```python
from build123d import *

# Parameters (mm, degrees)
SKETCH1_W               = 7
SKETCH1_H               = 15
BOSS_EXTRUDE1_DEPTH     = 9
SKETCH2_R               = 4.5
CUT_EXTRUDE1_DEPTH      = 14.647344064
CUT_EXTRUDE2_DEPTH      = 2.1
CUT_EXTRUDE2_DEPTH_BACK = 2.1
SKETCH3_R               = 6.1
FILLET1_R               = 7.5
BOSS_EXTRUDE2_DEPTH     = 4
SKETCH5_R               = 1.75
CUT_EXTRUDE3_DEPTH      = 17.194134741


with BuildPart() as part:
    # Sketch1 → Boss-Extrude1 (new body)
    with BuildSketch(Plane.XY):
        Rectangle(SKETCH1_W, SKETCH1_H)
    extrude(amount=BOSS_EXTRUDE1_DEPTH)

    # Sketch2 → Cut-Extrude1 (cut, through all)
    with BuildSketch(Plane(origin=(3.5, 0, 0), x_dir=(0, 0, -1), z_dir=(1, 0, 0))):
        Circle(SKETCH2_R)
    extrude(amount=-CUT_EXTRUDE1_DEPTH, mode=Mode.SUBTRACT)

    # Sketch3 → Cut-Extrude2 (cut, two sides: drawn at the far end of the back side and taken through both)
    with BuildSketch(Plane(origin=(0, 0, 0), x_dir=(0, 0, -1), z_dir=(1, 0, 0)).offset(-CUT_EXTRUDE2_DEPTH_BACK)):
        Circle(SKETCH3_R)
    extrude(amount=CUT_EXTRUDE2_DEPTH + CUT_EXTRUDE2_DEPTH_BACK, mode=Mode.SUBTRACT)

    # Fillet1
    fillet1_edges = [part.edges().sort_by_distance(p)[0] for p in [
        (0, -7.5, 9),
        (0, 7.5, 9),
    ]]
    fillet(fillet1_edges, radius=FILLET1_R - 0.0001)  # a hair under: the kernel refuses the full size

    # Sketch4 → Boss-Extrude2 (add)
    with BuildSketch(Plane.XY):
        with BuildLine():
            Line((-3.5, 6.507281557), (-3.5, 9.5))
            ThreePointArc((-3.5, 9.5), (0, 13), (3.5, 9.5))
            Line((3.5, 9.5), (3.5, 6.507281557))
            Line((3.5, 6.507281557), (-3.5, 6.507281557))
        make_face()
    boss_extrude2 = extrude(amount=BOSS_EXTRUDE2_DEPTH)

    # Sketch5 → Cut-Extrude3 (cut, through all)
    with BuildSketch(Plane(origin=(0, 0, 0), x_dir=(-1, 0, 0), z_dir=(0, 0, -1))):
        with Locations((0, 10)):
            Circle(SKETCH5_R)
    cut_extrude3 = extrude(amount=-CUT_EXTRUDE3_DEPTH, mode=Mode.SUBTRACT)

    # Mirror1: Boss-Extrude2, Cut-Extrude3 across plane
    add(boss_extrude2.mirror(Plane.ZX))
    add(cut_extrude3.mirror(Plane.ZX), mode=Mode.SUBTRACT)


solid = part.part
```
Verification items for the finished model (mm, model axes). A direction names the side the tool comes from. Round coordinates to 2 decimals unless told otherwise and drop trailing zeros. Order: outer loops, then holes, each group sorted by start corner. A loop starts at its lowest first (then second) coordinate and runs counter-clockwise, first axis right, second up.
1) Cross-section at A-A, the plane x = 0. Give the number of separate pieces and of enclosed holes in the cut face, plus the area to 3 significant figures.
Geometry says:
separate pieces: 3
enclosed holes: 0
area: 69.1 mm2
2) Cross-section at B-B, the plane z = 3.25. Record the cut outline in (x, y).
Geometry says:
outline: (-3.5, -9.5) arc R3.5 ccw to (3.5, -9.5) - (3.5, -3.11) - (2.1, -3.11) - (2.1, -5.16) - (-2.1, -5.16) - (-2.1, -3.11) - (-3.5, -3.11) - close; (-3.5, 3.11) - (-2.1, 3.11) - (-2.1, 5.16) - (2.1, 5.16) - (2.1, 3.11) - (3.5, 3.11) - (3.5, 9.5) arc R3.5 ccw to (-3.5, 9.5) - close; hole circle Ø3.5 at (0, -10); hole circle Ø3.5 at (0, 10)
3) Depth check by flat-ended pin: pin 1 (3 mm diameter, centred on x = -2.5, z = 3, fed in from -Y). Enter the tip coordinate at first touch or a pass-through.
Geometry says:
pin 1: stops at y = -12.85
4) Cross-section at D-D, the plane y = -0.25. Record the cut outline in (x, z).
Geometry says:
outline: (-3.5, 4.49) - (-2.1, 4.49) - (-2.1, 6.09) - (2.1, 6.09) - (2.1, 4.49) - (3.5, 4.49) - (3.5, 9) - (-3.5, 9) - close
5) Material ranges on line 1 (Y direction, x = 0, z = 2.8); line 2 (Y direction, x = -1.5, z = 2); line 3 (Z direction, x = -2, y = -9), recorded low to high.
Geometry says:
line 1: y = -13 to -11.75, -8.25 to -5.42, 5.42 to 8.25, 11.75 to 13
line 2: y = -12.66 to -10.9, -9.1 to -5.76, 5.76 to 9.1, 10.9 to 12.66
line 3: z = 0 to 4
6) Draft check along X on faces 6 (the flat face through (-2.1, 1.44, 4.45)), 7 (the flat face through (0, 8, 0)), 8 (the flat face through (-3.5, 0, 5)). Enter one of: +X half, -X half, draft (parallel to the pull), parting line (faces both ways), or undercut.
Geometry says:
face 6: undercut
face 7: draft
face 8: -X half
7) Tool access check on faces 1 (the cylindrical face through (0.228, 11.735, 1.972)), 2 (the cylindrical face through (0, 13, 2)), 3 (the flat face through (0, -8, 4)), 4 (the flat face through (0, 8, 4)), 5 (the flat face through (2.1, 1.44, 4.45)). Record the directions out of +Z, -Z, +X, -X, +Y, -Y that give a thin tool (end or side, any length) a straight path to the whole face; none if there is none.
Geometry says:
face 1: +Z, -Z
face 2: +Z, -Z, +Y
face 3: +Z, +X, -X, -Y
face 4: +Z, +X, -X, +Y
face 5: -Z
8) Cross-section at C-C, the plane y = 10. Record the cut outline in (x, z).
Geometry says:
outline: (-3.46, 0) - (-1.75, 0) - (-1.75, 4) - (-3.46, 4) - close; (1.75, 0) - (3.46, 0) - (3.46, 4) - (1.75, 4) - close
